CAD build for the part. Positions are in the model's coordinates, mm. A direction names the side the tool comes from. Round coordinates to 2 decimals unless told otherwise and drop trailing zeros. Write each loop counter-clockwise with the first axis right and the second up, starting at its lowest first coordinate (ties: lowest second). Pieces come first, ordered by that corner, then holes. Notation, with made-up numbers: (15, 16) - (40, 16) arc R23 ccw to (40, 29) - close; hole circle Ø3 at (51, -22). An arc over 180 degrees is marked (long way). Put each result on its own line as item: value. Start each with the question number.
Item 1: Cut at D-D (x = -10.5). Give the cut face in (y, z), and give its area (3 significant figures).
Item 2: Pin check, flat tips, straight feed: pin 1 Ø10 at (y, z) = (9.5, 5.5) entering from -X; pin 2 Ø4 at (y, z) = (2.5, -4.5) entering from -X; pin 3 Ø1.4 at (x, y) = (30.25, 2.75) entering from +Z; pin 4 Ø10 at (y, z) = (10.5, 1.5) entering from +X. Stop position of each tip, or through.
Item 3: Mould opens along X. For faces 1 (the flat face through (30, 6, -8.25)), 2 (the cylindrical face through (-25.65, 10.14, 14.68)), 3 (the flat face through (24.25, 10, -1)) say: released by +X, released by -X, zero draft, split by the parting line, or undercut.
Item 4: Cut at A-A (z = -10.5). Give the cut face in (x, y).
Item 5: Cut at C-C (z = -7.5). Give the cut face in (x, y), and give its area (3 significant figures).
Item 6: Drill centre lines: line 1 (X direction, y = 3.25, z = 10); line 2 (Z direction, x = 14, y = 2); line 3 (Y direction, x = 30.25, z = -11.65). Where is each one in solid material? Low to high. Write a range as from..to.
Item 7: 3-axis set-ups, long thin cutter, end or side, ignore diameter. For faces 4 (the flat face through (0, 0, 14)), 5 (the flat face through (-26.25, 10, 4)), 6 (the flat face through (-24.25, 10, -1)): which of +Z, -Z, +X, -X, +Y, -Y reach the whole face in a straight line?
Item 8: Cut at B-B (y = 2.75). Give the cut face in (x, z).
```python
from build123d import *

# Parameters (mm, degrees)
BOSS_EXTRUDE1_DEPTH = 20
FILLET1_R           = 2
SKETCH2_R           = 0.75
BOSS_EXTRUDE2_DEPTH = 5
FILLET2_R           = 2


with BuildPart() as part:
    # Sketch1 → Boss-Extrude1 (new body)
    with BuildSketch(Plane(origin=(0, 0, 0), x_dir=(1, 0, 0), z_dir=(0, 1, 0))):
        Polygon((26.25, 13.25), (26.25, -15.25), (-26.25, -15.25), (-26.25, 13.25), (-24.25, 13.25), (-24.25, -13.25), (24.25, -13.25), (24.25, 13.25), align=None)
    extrude(amount=BOSS_EXTRUDE1_DEPTH)

    # Fillet1
    fillet1_edges = [part.edges().sort_by_distance(p)[0] for p in [
        (-24.25, 10, 13.25),
        (24.25, 10, 13.25),
        (26.25, 10, 15.25),
        (-26.25, 10, 15.25),
    ]]
    fillet(fillet1_edges, radius=FILLET1_R)

    # Sketch2 → Boss-Extrude2 (add)
    with BuildSketch(Plane(origin=(0, 0, -13.25), x_dir=(-1, 0, 0), z_dir=(0, 0, -1))):
        with BuildLine():
            Line((-26.25, 0), (-30.25, 0))
            ThreePointArc((-30.25, 0), (-32.529711414, 1.212009145), (-32.799945678, 3.779697548))
            Line((-32.799945678, 3.779697548), (-26.25, 20))
            Line((-26.25, 20), (-26.25, 0))
        make_face()
        with Locations((-30.25, 2.75)):
            Circle(SKETCH2_R, mode=Mode.SUBTRACT)
    boss_extrude2 = extrude(amount=-BOSS_EXTRUDE2_DEPTH)

    # Mirror1: Boss-Extrude2 across plane
    add(boss_extrude2.mirror(Plane(origin=(0, 0, 0), x_dir=(0, 0, 1), z_dir=(1, 0, 0))))

    # Fillet2
    fillet2_edges = [part.edges().sort_by_distance(p)[0] for p in [
        (26.25, 10, -8.25),
        (-26.25, 10, -8.25),
    ]]
    fillet(fillet2_edges, radius=FILLET2_R)


solid = part.part
```
Output values:
1. outline: (0, 13.25) - (20, 13.25) - (20, 15.25) - (0, 15.25) - close
1. area: 40.0 mm2
2. pin 1: x = -26.25
2. pin 2: x = -26.27
2. pin 3: through
2. pin 4: x = 26.25
3. face 1: zero draft
3. face 2: released by -X
3. face 3: undercut
4. outline: (-32.8, 3.78) arc R2.75 ccw to (-30.25, 0) - (-24.25, 0) - (-24.25, 20) - (-26.25, 20) - close; (24.25, 0) - (30.25, 0) arc R2.75 ccw to (32.8, 3.78) - (26.25, 20) - (24.25, 20) - close; hole circle Ø1.5 at (-30.25, 2.75); hole circle Ø1.5 at (30.25, 2.75)
5. outline: (-26.69, 0) - (-24.25, 0) - (-24.25, 20) - (-26.25, 20) - (-26.69, 18.91) - close; (24.25, 0) - (26.69, 0) - (26.69, 18.91) - (26.25, 20) - (24.25, 20) - close
5. area: 97.1 mm2
6. line 1: -26.25..-24.25, 24.25..26.25
6. line 2: 13.25..15.25
6. line 3: 0..2, 3.5..10.09
7. face 4: +Z, -Z, +X, -X, -Y
7. face 5: +Z, -X, +Y, -Y
7. face 6: -Z, +Y, -Y
8. outline: (-33, -13.25) - (-31, -13.25) - (-31, -8.25) - (-33, -8.25) - close; (-29.5, -13.25) - (-24.25, -13.25) - (-24.25, 11.25) arc R2 cw to (-22.25, 13.25) - (22.25, 13.25) arc R2 cw to (24.25, 11.25) - (24.25, -13.25) - (29.5, -13.25) - (29.5, -8.25) - (28.25, -8.25) arc R2 cw to (26.25, -6.25) - (26.25, 13.25) arc R2 ccw to (24.25, 15.25) - (-24.25, 15.25) arc R2 ccw to (-26.25, 13.25) - (-26.25, -6.25) arc R2 cw to (-28.25, -8.25) - (-29.5, -8.25) - close; (31, -13.25) - (33, -13.25) - (33, -8.25) - (31, -8.25) - close
